from build123d import *

# Parameters (mm, degrees)
SKETCH2_W       = 4
SKETCH2_H       = 0.6
SLOT_DEPTH      = 1.42
THDSCHPAT_COUNT = 14
THDSCHPAT_PITCH = 0.680345237


with BuildPart() as part:
    # BodySke → BaseBody (revolve)
    with BuildSketch(Plane.XY):
        Polygon((9.75, 1.25), (12, 1.25), (12, 0), (0, 0), (0, 1.61), (0.225166605, 2), (9, 2), align=None)
    revolve(axis=Axis((-12.7, 0, 0), (1, 0, 0)))

    # Sketch2 → Slot (cut)
    with BuildSketch(Plane(origin=(0, 0, 0), x_dir=(0, 0, -1), z_dir=(1, 0, 0))):
        Rectangle(SKETCH2_W, SKETCH2_H)
    extrude(amount=SLOT_DEPTH, mode=Mode.SUBTRACT)

    # ThdSchSke → ThreadSchematic (revolve, cut)
    with BuildSketch(Plane.XY):
        Polygon((0.225166605, -1.61), (-0.047914335, -2), (-0.047914335, -2.5), (0.498247545, -2.5), (0.498247545, -2), align=None)
    threadschematic = revolve(axis=Axis((-3.175, 0, 0), (1, 0, 0)), mode=Mode.SUBTRACT)

    # ThdSchPat: ThreadSchematic ×14
    with Locations(*[(i * THDSCHPAT_PITCH, 0, 0) for i in range(1, THDSCHPAT_COUNT)]):
        add(threadschematic, mode=Mode.SUBTRACT)


solid = part.part
Source: CAD feature listing. Evaluate the final solid. Frame: model axes, mm. Coordinates: 2 decimals unless noted, no trailing zeros. Loops run counter-clockwise (first coordinate to the right, second up) from the corner with the lowest first, then second, coordinate; pieces in that order, holes last. Notation, with made-up numbers: (51, 30.25) - (81, 30.25) arc R25 ccw to (81, 42.25) - close; hole circle Ø4 at (0.5, 66). An arc over 180 degrees is marked (long way). One line per question, with ' | ' between items.
1) First-contact query: P1, Ø0.5, axis at y = 0, z = 0.5, coming from the -X side; P2, Ø1, axis at x = 6.5, y = 0, coming from the +Z side; P3, Ø0.7, axis at x = 0.5, z = -1, coming from the +Y side. Flat tips, straight axial feed; report the tip coordinate or a pass-through.
Report:
P1: stops at x = 1.42 | P2: stops at z = 2 | P3: stops at y = 1.89
2) Section A-A, the plane x = 3.5. Return loops of the section in (y, z), then the cut area to 3 significant figures.
Report:
outline: circle Ø3.58 at (0, 0) | area: 10.1 mm²
3) Line query: line 1 along X through (y, z) = (-0.2, 0.75); line 2 along Z through (x, y) = (8.25, -0.2); line 3 along Y through (x, z) = (1, -0.7). Output: solid intervals per line, ascending.
Report:
line 1: x = 1.42 to 12 | line 2: z = -1.8 to 1.8 | line 3: y = -1.6 to -0.3, 0.3 to 1.6
4) Pull-direction query (X, two-part tool) for faces 1 (the face through (0.8, 1.76, -0.04)), 2 (the face through (1, 0.3, 0)); classes: released by +X, released by -X, zero draft, split by the parting line, or undercut.
Report:
face 1: undercut | face 2: zero draft
